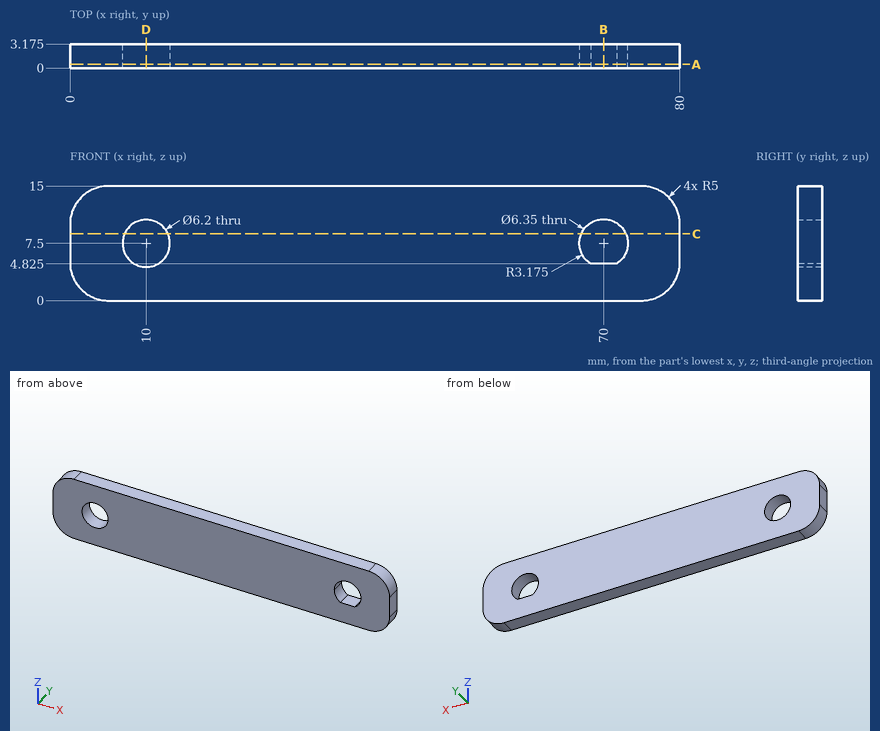
Print and shaded views of the part. All mm, measured from the part's lowest x, y and z. Give positions to 0.01 mm unless a question says otherwise; leave off trailing zeros. Write each loop counter-clockwise with the first axis right and the second up, starting at its lowest first coordinate (ties: lowest second). Pieces come first, ordered by that corner, then holes. Notation, with made-up numbers: (75, 17) -> (115, 17) arc R9 ccw to (115, 30) -> close; hole circle Ø11 at (22.25, 43). An arc over 180 degrees is marked (long way). Use CSV: the item, a comma, the result in double quotes. Start each with the question number.
1) Cut at D-D on x = 10. List the corners of the cut face in (y, z) (3 decimals).
2) Cut at A-A on y = 0.5. List the corners of the cut face in (x, z) (3 decimals).
3) Drill centre lines: L1, parallel to Z at x = 70, y = 1.1 (3 decimals); L2, parallel to X at y = 0.2, z = 5.75; L3, parallel to Z at x = 10, y = 0.7. Where is each one in solid material? Low to high.
4) Cut at B-B on x = 70. List the corners of the cut face in (y, z) (3 decimals).
5) Cut at C-C on z = 8.75. List the corners of the cut face in (x, y) (3 decimals), plus the area to 3 significant figures.
6) Pin check, flat tip, straight feed: P1, Ø5, axis at x = 10, z = 7.5, coming from the -Y side. Stop position of the tip, or through.
Final values:
1,outline,"(0, 0) -> (3.175, 0) -> (3.175, 4.4) -> (0, 4.4) -> close; (0, 10.6) -> (3.175, 10.6) -> (3.175, 15) -> (0, 15) -> close"
2,outline,"(0, 5) arc R5 ccw to (5, 0) -> (75, 0) arc R5 ccw to (80, 5) -> (80, 10) arc R5 ccw to (75, 15) -> (5, 15) arc R5 ccw to (0, 10) -> close; hole circle Ø6.2 at (10, 7.5); hole (66.825, 7.5) arc R3.175 ccw to (68.29, 4.825) -> (71.71, 4.825) arc R3.175 ccw (long way) to start"
3,L1,"z = 0 to 4.825, 10.675 to 15"
3,L2,"x = 0 to 7.44, 12.56 to 67.35, 72.65 to 80"
3,L3,"z = 0 to 4.4, 10.6 to 15"
4,outline,"(0, 0) -> (3.175, 0) -> (3.175, 4.825) -> (0, 4.825) -> close; (0, 10.675) -> (3.175, 10.675) -> (3.175, 15) -> (0, 15) -> close"
5,outline,"(0, 0) -> (7.163, 0) -> (7.163, 3.175) -> (0, 3.175) -> close; (12.837, 0) -> (67.081, 0) -> (67.081, 3.175) -> (12.837, 3.175) -> close; (72.919, 0) -> (80, 0) -> (80, 3.175) -> (72.919, 3.175) -> close"
5,area,"217 mm2"
6,P1,"passes through"
